```python
from build123d import *

# Parameters (mm, degrees)
SKETCH1_W           = 3
SKETCH1_H           = 24
BOSS_EXTRUDE1_DEPTH = 23
SKETCH2_W           = 6
SKETCH2_H           = 24
BOSS_EXTRUDE2_DEPTH = 2
SKETCH4_W           = 3
SKETCH4_H           = 24
BOSS_EXTRUDE3_DEPTH = 2
SKETCH5_W           = 24
SKETCH5_H           = 27
CUT_EXTRUDE1_DEPTH  = 0.5


with BuildPart() as part:
    # Sketch1 → Boss-Extrude1 (new body)
    with BuildSketch(Plane(origin=(0, 0, 0), x_dir=(1, 0, 0), z_dir=(0, 1, 0))):
        with Locations((1.5, 12)):
            Rectangle(SKETCH1_W, SKETCH1_H)
    extrude(amount=BOSS_EXTRUDE1_DEPTH)

    # Sketch2 → Boss-Extrude2 (add)
    with BuildSketch(Plane(origin=(0, 23, 0), x_dir=(1, 0, 0), z_dir=(0, 1, 0))):
        with Locations((0, 12)):
            Rectangle(SKETCH2_W, SKETCH2_H)
    extrude(amount=BOSS_EXTRUDE2_DEPTH)

    # Sketch4 → Boss-Extrude3 (add)
    with BuildSketch(Plane.XZ):
        with Locations((1.5, -12)):
            Rectangle(SKETCH4_W, SKETCH4_H)
    extrude(amount=BOSS_EXTRUDE3_DEPTH)

    # Sketch5 → Cut-Extrude1 (cut)
    with BuildSketch(Plane(origin=(3, 0, 0), x_dir=(0, 0, -1), z_dir=(1, 0, 0))):
        with Locations((12, 11.5)):
            Rectangle(SKETCH5_W, SKETCH5_H)
    extrude(amount=-CUT_EXTRUDE1_DEPTH, mode=Mode.SUBTRACT)


solid = part.part
```
Verification items for the finished model (mm, model axes). A direction names the side the tool comes from. Round coordinates to 2 decimals unless told otherwise and drop trailing zeros. Write each loop counter-clockwise with the first axis right and the second up, starting at its lowest first coordinate (ties: lowest second). Pieces come first, ordered by that corner, then holes. Notation, with made-up numbers: (59.25, -30) - (92.25, -30) arc R17 cw to (92.25, -5) - close; hole circle Ø9 at (-3.75, 51.5). An arc over 180 degrees is marked (long way). Answer as a JSON object with one key per item and string values. Group by question number.
Q1. Go/stop test with flat-tipped pins: pin 1 Ø2.5 at (x, z) = (-2, -14.5) entering from -Y; pin 2 Ø3 at (x, y) = (-2, 9.5) entering from -Z; pin 3 Ø7 at (y, z) = (5.5, -9) entering from -X. Record where each tip stops, or that it passes through.
Q2. Thickness scan on line 1 (X direction, y = 8, z = -2); line 2 (Y direction, x = -1.3, z = -14). Record the ranges inside material, lowest first.
Q3. Section check B-B, the plane y = 3.5. Enter the section's corners in (x, z), plus the area to 3 significant figures.
Q4. Tool access check on faces 1 (the flat face through (0, 11, -12)), 2 (the flat face through (1, 12, 0)). Record the directions out of +Z, -Z, +X, -X, +Y, -Y that give a thin tool (end or side, any length) a straight path to the whole face; none if there is none.
Q5. Section check A-A, the plane z = -11.5. Enter the section's corners in (x, y).
Q6. Section check C-C, the plane x = -1.45. Enter the section's corners in (y, z).
Found:
{
 "1": {"pin 1": "stops at y = 23", "pin 2": "passes through", "pin 3": "stops at x = 0"},
 "2": {"line 1": "x = 0 to 2.5", "line 2": "y = 23 to 25"},
 "3": {"outline": "(0, -24) - (2.5, -24) - (2.5, 0) - (0, 0) - close", "area": "60.0 mm^2"},
 "4": {"face 1": "+Z, -Z, -X, -Y", "face 2": "+Z, +X, -X, +Y, -Y"},
 "5": {"outline": "(-3, 23) - (0, 23) - (0, -2) - (2.5, -2) - (2.5, 25) - (-3, 25) - close"},
 "6": {"outline": "(23, -24) - (25, -24) - (25, 0) - (23, 0) - close"}
}
